The model under review builds one solid part; all positions refer to its coordinate system, in mm. Face numbers are marked on the shaded views. A direction names the side the tool comes from. Give positions to 0.01 mm unless a question says otherwise; leave off trailing zeros. Loops run counter-clockwise (first coordinate to the right, second up) from the corner with the lowest first, then second, coordinate; pieces in that order, holes last. Notation, with made-up numbers: M 49.5,33.25 L 92.5,33.25 A27 ccw 92.5,65.25 Z; hole C 0,-25 d11. An arc over 180 degrees is marked long. Return JSON: item names as keys, results as strings.
```python
from build123d import *

# Parameters (mm, degrees)
SKETCH_3_W          = 26
SKETCH_3_H          = 36
EXTRUDE_1_DEPTH     = 4
CUT_EXTRUDE_1_REACH = 24.561
SKETCH_4_R          = 1.7
SKETCH_5_W          = 26
SKETCH_5_H          = 4
EXTRUDE_2_DEPTH     = 14


with BuildPart() as part:
    # Эскиз3 → Бобышка-Вытянуть1 (new body)
    with BuildSketch(Plane.XY):
        Rectangle(SKETCH_3_W, SKETCH_3_H)
    extrude(amount=EXTRUDE_1_DEPTH)

    # Эскиз4 → Вырез-Вытянуть1 (cut, up to next)
    with BuildSketch(Plane.XY.offset(4), mode=Mode.PRIVATE) as cut_extrude_1_sk1:
        with Locations((-7, -11)):
            Circle(SKETCH_4_R)
    cut_extrude_1_tool1 = extrude(cut_extrude_1_sk1.sketch, amount=-CUT_EXTRUDE_1_REACH, mode=Mode.PRIVATE) & part.part
    # Эскиз4 → Вырез-Вытянуть1 (cut, up to next)
    with BuildSketch(Plane.XY.offset(4), mode=Mode.PRIVATE) as cut_extrude_1_sk2:
        with Locations(Location((7, -11, 0), (0, 0, 180))):
            Circle(SKETCH_4_R)
    cut_extrude_1_tool2 = extrude(cut_extrude_1_sk2.sketch, amount=-CUT_EXTRUDE_1_REACH, mode=Mode.PRIVATE) & part.part
    add(cut_extrude_1_tool1.solids().sort_by_distance((-7, -11, 4))[0], mode=Mode.SUBTRACT)
    add(cut_extrude_1_tool2.solids().sort_by_distance((7, -11, 4))[0], mode=Mode.SUBTRACT)

    # Эскиз5 → Бобышка-Вытянуть2 (add)
    with BuildSketch(Plane.XY.offset(4)):
        with Locations((0, 16)):
            Rectangle(SKETCH_5_W, SKETCH_5_H)
    extrude(amount=EXTRUDE_2_DEPTH)


solid = part.part
```
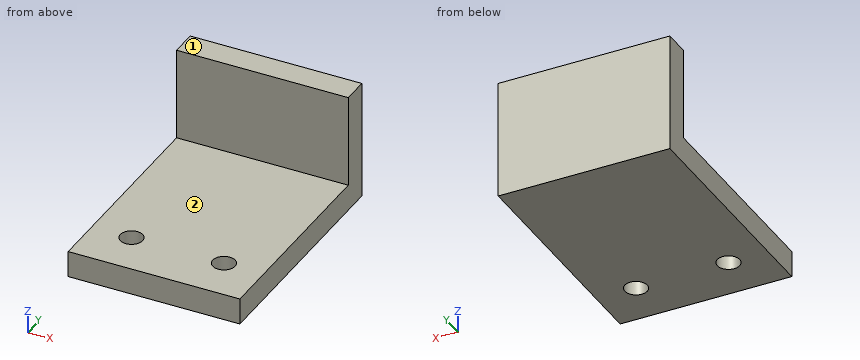
1) Consider section C-C on z = 1.5. Write out the cut boundary in (x, y), then the cut area to 3 significant figures.
From the geometry:
{"outline": "M -13,-18 L 13,-18 L 13,18 L -13,18 Z; hole C -7,-11 d3.4; hole C 7,-11 d3.4", "area": "918 mm²"}
2) Wall thickness on L1, parallel to Y at x = -7, z = 1.75; L2, parallel to Y at x = 1.75, z = 7.75; L3, parallel to Z at x = -4.25, y = -9: over which ranges is each line inside the solid? List them lowest first. Write a range as from..to.
From the geometry:
{"L1": "-18..-12.7, -9.3..18", "L2": "14..18", "L3": "0..4"}
3) Consider section D-D on x = -10.75. Write out the cut boundary in (y, z), then the cut area to 3 significant figures.
From the geometry:
{"outline": "M -18,0 L 18,0 L 18,18 L 14,18 L 14,4 L -18,4 Z", "area": "200 mm²"}
4) Consider section A-A on x = 7. Write out the cut boundary in (y, z), then the cut area to 3 significant figures.
From the geometry:
{"outline": "M -18,0 L -12.7,0 L -12.7,4 L -18,4 Z; M -9.3,0 L 18,0 L 18,18 L 14,18 L 14,4 L -9.3,4 Z", "area": "186 mm²"}
5) Consider section B-B on y = -11. Write out the cut boundary in (x, z).
From the geometry:
{"outline": "M -13,0 L -8.7,0 L -8.7,4 L -13,4 Z; M -5.3,0 L 5.3,0 L 5.3,4 L -5.3,4 Z; M 8.7,0 L 13,0 L 13,4 L 8.7,4 Z"}
6) Insertion check: pin 1 (5 mm diameter, centred on x = 2, y = -8, fed in from +Z); pin 2 (10 mm diameter, centred on x = -4, z = 11, fed in from -Y). Each pin has a flat end and moves straight along its axis. Give the tip position at first contact, or say it passes through.
From the geometry:
{"pin 1": "z = 4", "pin 2": "y = 14"}
7) Tool access review of the marked faces 1 and 2: name each direction out of +Z, -Z, +X, -X, +Y, -Y from which nothing blocks a thin tool from reaching the whole face with its end or side.
From the geometry:
{"face 1": "+Z, +X, -X, +Y, -Y", "face 2": "+Z, +X, -X, -Y"}
